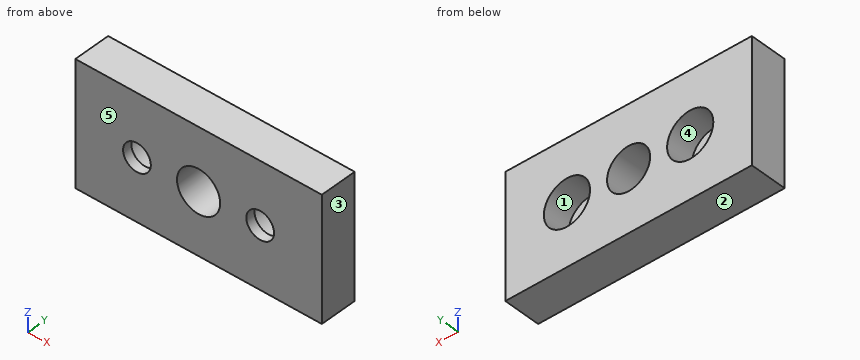
```python
from build123d import *

# Parameters (mm, degrees)
SKETCH_1_W             = 80
SKETCH_1_H             = 40
EXTRUDE_1_DEPTH        = 12
HOLE_WIZARD_M161_D     = 14
HOLE_WIZARD_M161_DEPTH = 12


with BuildPart() as part:
    # Эскиз1 → Бобышка-Вытянуть1 (new body)
    with BuildSketch(Plane(origin=(0, 0, 0), x_dir=(1, 0, 0), z_dir=(0, 1, 0))):
        Rectangle(SKETCH_1_W, SKETCH_1_H)
    extrude(amount=EXTRUDE_1_DEPTH)

    # Эскиз2 → Вырез-Повернуть1 (revolve, cut)
    with BuildSketch(Plane.XY):
        Polygon((-27.5, 12), (-27.5, 3), (-24.5, 3), (-24.5, 0), (-20, 0), (-20, 12), align=None)
    cut_revolve_1 = revolve(axis=Axis((-20, 12, 0), (0, -1, 0)), mode=Mode.SUBTRACT)

    # Зеркальное отражение1: Вырез-Повернуть1 across plane
    add(cut_revolve_1.mirror(Plane(origin=(0, 0, 0), x_dir=(0, 0, 1), z_dir=(1, 0, 0))), mode=Mode.SUBTRACT)

    # Отверстие обработанное метчиком M161
    with Locations(Plane(origin=(0, 12, 0), x_dir=(1, 0, 0), z_dir=(0, 1, 0))):
        with Locations((0, 0)):
            Hole(HOLE_WIZARD_M161_D / 2, depth=HOLE_WIZARD_M161_DEPTH)


solid = part.part
```
Input: part model. Units: mm. Frame: model coordinates. Face numbers are marked on the shaded views. A direction names the side the tool comes from. Coordinates: 2 decimals unless noted, no trailing zeros. Loops run counter-clockwise (first coordinate to the right, second up) from the corner with the lowest first, then second, coordinate; pieces in that order, holes last. Notation, with made-up numbers: M 66,11 L 93,11 A14 cw 93,20 Z; hole C 11.25,9.25 d6. An arc over 180 degrees is marked long. Use a Markdown table: item, result. Add a question column.
1) Section D-D, the plane x = 14. Return the cut outline in (y, z).
2) Section A-A, the plane y = 7.5. Return the cut outline in (x, z), plus the area to 3 significant figures.
3) Set-up query: the marked faces 4 and 5. Return all of +Z, -Z, +X, -X, +Y, -Y with unobstructed straight access to the full face (end or side cutting, diameter ignored); none if empty.
4) Pin query (flat end, axial travel): P1, Ø7.5, axis at x = 18, z = -1.5, coming from the +Y side; P2, Ø7, axis at x = 20, z = 0, coming from the -Y side. Return the tip coordinate at first contact, or that it passes through.
5) Section B-B, the plane x = -20. Return the cut outline in (y, z), plus the area to 3 significant figures.
6) Section C-C, the plane z = 2. Return the cut outline in (x, y), plus the area to 3 significant figures.
7) Draft query along X for the marked faces 1, 2 and 3. Return one class per face: +X half, -X half, draft (parallel to the pull), parting line (faces both ways), or undercut.
8) Line query: L1, parallel to Z at x = 0, y = 5.5; L2, parallel to Z at x = -20, y = 10; L3, parallel to X at y = 5.75, z = -5.5. Output: solid intervals per line, ascending. Write a range as from..to.
Answer below:
| question | item | result |
|---|---|---|
| 1 | outline | M 0,-20 L 12,-20 L 12,-4.5 L 3,-4.5 L 3,4.5 L 12,4.5 L 12,20 L 0,20 Z |
| 2 | outline | M -40,-20 L 40,-20 L 40,20 L -40,20 Z; hole C -20,0 d15; hole C 0,0 d14; hole C 20,0 d15 |
| 2 | area | 2,690 mm2 |
| 3 | face 4 | +Y |
| 3 | face 5 | +Z, -Z, +X, -X, -Y |
| 4 | P1 | y = 3 |
| 4 | P2 | through |
| 5 | outline | M 0,-20 L 12,-20 L 12,-7.5 L 3,-7.5 L 3,-4.5 L 0,-4.5 Z; M 0,4.5 L 3,4.5 L 3,7.5 L 12,7.5 L 12,20 L 0,20 Z |
| 5 | area | 318 mm2 |
| 6 | outline | M -40,0 L -24.03,0 L -24.03,3 L -27.23,3 L -27.23,12 L -40,12 Z; M -15.97,0 L -6.71,0 L -6.71,12 L -12.77,12 L -12.77,3 L -15.97,3 Z; M 6.71,0 L 15.97,0 L 15.97,3 L 12.77,3 L 12.77,12 L 6.71,12 Z; M 24.03,0 L 40,0 L 40,12 L 27.23,12 L 27.23,3 L 24.03,3 Z |
| 6 | area | 490 mm2 |
| 7 | face 1 | undercut |
| 7 | face 2 | draft |
| 7 | face 3 | +X half |
| 8 | L1 | -20..-7, 7..20 |
| 8 | L2 | -20..-7.5, 7.5..20 |
| 8 | L3 | -40..-25.1, -14.9..-4.33, 4.33..14.9, 25.1..40 |
